The listing builds one solid part. Answer for the finished solid, in the listing's coordinates (mm). A direction names the side the tool comes from. Coordinates: 2 decimals unless noted, no trailing zeros. Order: outer loops, then holes, each group sorted by start corner. A loop starts at its lowest first (then second) coordinate and runs counter-clockwise, first axis right, second up. Notation, with made-up numbers: (-14, 84.5) -> (44, 84.5) arc R20 ccw to (44, 111.5) -> close; hole circle Ø7 at (81, 16.5). An arc over 180 degrees is marked (long way). Return JSON: item names as keys, results as strings.
```python
from build123d import *

# Parameters (mm, degrees)
F0_W     = 130
F0_H     = 108
F1_DEPTH = 45
F2_W     = 108
F2_H     = 25
F3_DEPTH = 47
F4_W     = 25
F4_H     = 50
F5_DEPTH = 70.001


with BuildPart() as f1:
    # F0 (on Top) → F1 (new body)
    with BuildSketch(Plane.XY):
        Rectangle(F0_W, F0_H)
    extrude(amount=F1_DEPTH)

    # F2 (on face) → F3 (join)
    with BuildSketch(Plane(origin=(-65, 0, 0), x_dir=(0, -1, 0), z_dir=(-1, 0, 0))):
        with Locations((0, 57.5)):
            Rectangle(F2_W, F2_H)
    extrude(amount=-F3_DEPTH)

    # F4 (on face) → F5 (cut, through all)
    with BuildSketch(Plane.XY.offset(70)):
        with Locations((-52.5, 0)):
            Rectangle(F4_W, F4_H)
    extrude(amount=-F5_DEPTH, mode=Mode.SUBTRACT)


solid = f1.part
```
Item 1: Find the intervals of material crossed by probe 1 along Y at (x, z) = (-60, 35.5); probe 2 along Z at (x, y) = (0.5, 42); probe 3 along X at (y, z) = (-20.5, 53), in increasing order.
Answer list:
{"probe 1": "-54 to -25, 25 to 54", "probe 2": "0 to 45", "probe 3": "-40 to -18"}
Item 2: The part is cut by section A-A on x = -48.5. Determine the outline of the cut face in (y, z), plus the area to 3 significant figures.
Answer list:
{"outline": "(-54, 0) -> (-25, 0) -> (-25, 70) -> (-54, 70) -> close; (25, 0) -> (54, 0) -> (54, 70) -> (25, 70) -> close", "area": "4,060 mm2"}
Item 3: The part is cut by section D-D on x = 41.5. Determine the outline of the cut face in (y, z), plus the area to 3 significant figures.
Answer list:
{"outline": "(-54, 0) -> (54, 0) -> (54, 45) -> (-54, 45) -> close", "area": "4,860 mm2"}
Item 4: The part is cut by section B-B on z = 50.5. Determine the outline of the cut face in (x, y).
Answer list:
{"outline": "(-65, -54) -> (-18, -54) -> (-18, 54) -> (-65, 54) -> (-65, 25) -> (-40, 25) -> (-40, -25) -> (-65, -25) -> close"}
Item 5: Determine the mould class of faces 4 (the flat face through (65, -1, 22)), 5 (the flat face through (-53, 25, 35)), 6 (the flat face through (-1, 54, 27)) for opening direction Y: pulls with the +Y half, pulls with the -Y half, needs draft (parallel to the pull), parting line crosses it, or undercut.
Answer list:
{"face 4": "needs draft", "face 5": "undercut", "face 6": "pulls with the +Y half"}
Item 6: Flat-ended cylindrical pins translate along their axes: pin 1 (20 mm diameter, centred on y = -25, z = 57, fed in from +X); pin 2 (25 mm diameter, centred on y = -1, z = 30, fed in from -X). Find the tip coordinate at first contact, or state that the pin passes through.
Answer list:
{"pin 1": "x = -18", "pin 2": "x = -40"}
Item 7: Which of the six approach directions +Z, -Z, +X, -X, +Y, -Y give full straight-line access (tool end or side, diameter ignored) to faces 1 (the flat face through (-53, -25, 35)), 2 (the flat face through (-37, 1, 70)), 3 (the flat face through (23, 1, 45))?
Answer list:
{"face 1": "+Z, -Z, -X", "face 2": "+Z, +X, -X, +Y, -Y", "face 3": "+Z, +X, +Y, -Y"}
Item 8: The part is cut by section C-C on y = 33.5. Determine the outline of the cut face in (x, z).
Answer list:
{"outline": "(-65, 0) -> (65, 0) -> (65, 45) -> (-18, 45) -> (-18, 70) -> (-65, 70) -> close"}
